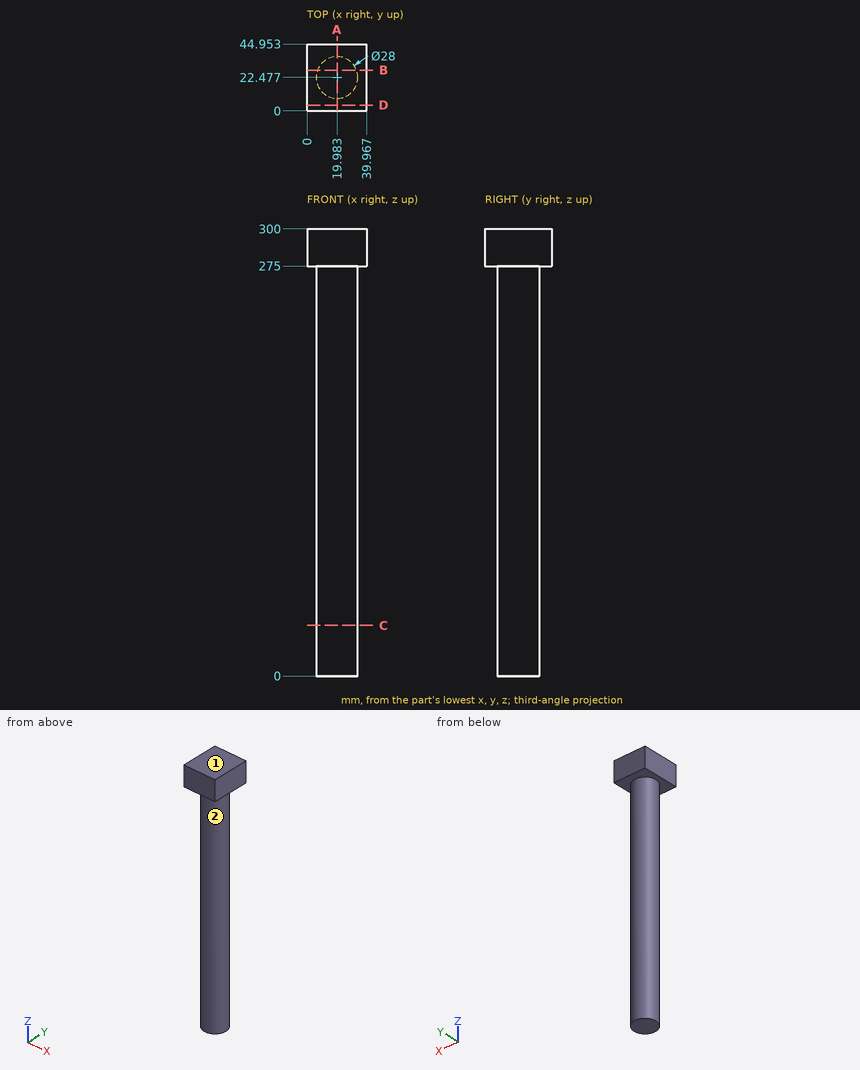
Can you work these out from the drawing? Everything is in mm from the part's minimum corner. A direction names the side the tool comes from. Give positions to 0.01 mm unless a question says otherwise; leave off trailing zeros. Loops run counter-clockwise (first coordinate to the right, second up) from the corner with the lowest first, then second, coordinate; pieces in that order, holes last. Notation, with made-up numbers: (30.5, 88.5) -> (51.5, 88.5) arc R17 cw to (51.5, 112.5) -> close; hole circle Ø8 at (21.25, 9). An arc over 180 degrees is marked (long way). Write item = value, one per line.
1) Suppose I cut it at D-D on y = 4. Write out the boundary of the cut face in (x, z), then the cut area to 3 significant figures.
Check result:
outline = (0, 275) -> (39.97, 275) -> (39.97, 300) -> (0, 300) -> close
area = 999 mm2
2) For the marked faces 1 and 2, which set-ups out of +Z, -Z, +X, -X, +Y, -Y let a thin tool reach every point of the face, with its end or its side?
Check result:
face_1 = +Z, +X, -X, +Y, -Y
face_2 = -Z
3) Suppose I cut it at A-A on x = 20. Write out the boundary of the cut face in (y, z).
Check result:
outline = (0, 275) -> (8.48, 275) -> (8.48, 0) -> (36.48, 0) -> (36.48, 275) -> (44.95, 275) -> (44.95, 300) -> (0, 300) -> close
4) Will these pins go through, and if not, where does the flat tip stop? pin 1 (4 mm diameter, centred on y = 27.5, z = 53, fed in from -X); pin 2 (1 mm diameter, centred on x = 31.5, z = 205, fed in from +Y) (1 decimal); pin 3 (8 mm diameter, centred on x = 22.5, z = 246.5, fed in from +Y); pin 4 (8 mm diameter, centred on x = 17, y = 16.5, fed in from -Z).
Check result:
pin_1 = 6.31
pin_2 = 31.1
pin_3 = 36.48
pin_4 = 0
5) I need wall thicknesses on L1, parallel to Z at x = 10, y = 41; L2, parallel to Y at x = 19.5, z = 91.5 (1 decimal); L3, parallel to X at y = 21.5, z = 137.5. Which ranges of each line are inside material? Lowest first, please. Write a range as from..to.
Check result:
L1 = 275..300
L2 = 8.5..36.5
L3 = 6.02..33.95
6) Suppose I cut it at B-B on y = 27.5. Write out the boundary of the cut face in (x, z) (1 decimal).
Check result:
outline = (0, 275) -> (6.9, 275) -> (6.9, 0) -> (33.1, 0) -> (33.1, 275) -> (40, 275) -> (40, 300) -> (0, 300) -> close
7) Suppose I cut it at C-C on z = 34. Write out the boundary of the cut face in (x, y), then the cut area to 3 significant figures.
Check result:
outline = circle Ø28 at (19.98, 22.48)
area = 616 mm2
